Geometry: final body of the model. Coordinates: model frame, mm. A direction names the side the tool comes from. Round coordinates to 2 decimals unless told otherwise and drop trailing zeros. Loops run counter-clockwise (first coordinate to the right, second up) from the corner with the lowest first, then second, coordinate; pieces in that order, holes last. Notation, with made-up numbers: (-10.75, 31) - (22.25, 31) arc R25 cw to (22.25, 49) - close; hole circle Ø7 at (-14, -24). An arc over 180 degrees is marked (long way). Answer as a JSON object with one key per item and string values. Group by question number.
Item 1: Section A-A (x = -18.5). Return the cut outline in (y, z).
Item 2: Section C-C (y = 56). Return the cut outline in (x, z).
Item 3: Line query: line 1 (Z direction, x = -34, y = 81); line 2 (X direction, y = 6, z = 275.5); line 3 (Y direction, x = -4, z = 164.5). Output: solid intervals per line, ascending.
Item 4: Section B-B (z = 112.5). Return the cut outline in (x, y), plus the area to 3 significant figures.
Item 5: Draft query along Z for faces 1 (the face through (-6, 6, 0)), 2 (the face through (0, -7.94, 148)), 3 (the face through (0, 23, 267.65)). Return one class per face: released by +Z, released by -Z, zero draft, split by the parting line, or undercut.
Item 6: First-contact query: pin 1 (21 mm diameter, centred on x = -1.5, y = 23, fed in from -Z); pin 2 (2 mm diameter, centred on x = -12.5, y = 69.5, fed in from -Z); pin 3 (5.5 mm diameter, centred on x = 0, y = 31.94, fed in from -Z); pin 4 (1.2 mm diameter, centred on y = 17.5, z = 54.5, fed in from -X) (3 decimals). Flat tips, straight axial feed; report the tip coordinate or a pass-through.
Item 7: Reachability of faces 4 (the face through (0, 23, 51.38)), 5 (the face through (-6, -6, 0)), 6 (the face through (6, -6, 376)), 7 (the face through (0, 23, 174.38)) from +Z, -Z, +X, -X, +Y, -Y: full face, straight path, thin tool, end or side. Return the list, or none.
```python
from build123d import *

# Parameters (mm, degrees)
CROQUIS2_W              = 15.88
CROQUIS2_H              = 15.88
SALIENTE_EXTRUIR1_DEPTH = 300
CROQUIS3_R              = 7.94
SALIENTE_EXTRUIR2_DEPTH = 50
SALIENTE_EXTRUIR3_START = 50
CROQUIS5_R              = 7.94
SALIENTE_EXTRUIR3_DEPTH = 50
CROQUIS6_W              = 19.05
CROQUIS6_H              = 4
CROQUIS6_H_2            = 3.052323646
SALIENTE_EXTRUIR4_DEPTH = 30
CORTAR_EXTRUIR1_REACH   = 303.171
CROQUIS7_R              = 3
CROQUIS8_R              = 7.94
SALIENTE_EXTRUIR5_DEPTH = 30
CROQUIS9_R              = 15.735705631
SALIENTE_EXTRUIR6_DEPTH = 4


with BuildPart() as part:
    # Croquis2 → Saliente-Extruir1 (new body)
    with BuildSketch(Plane.XY):
        Rectangle(CROQUIS2_W, CROQUIS2_H)
    extrude(amount=SALIENTE_EXTRUIR1_DEPTH)

    # Croquis3 → Saliente-Extruir2 (add)
    with BuildSketch(Plane.XY.offset(300)):
        Circle(CROQUIS3_R)
    extrude(amount=SALIENTE_EXTRUIR2_DEPTH)

    # Croquis5 → Saliente-Extruir3 (add)
    with BuildSketch(Plane(origin=(0, 0, 0), x_dir=(-1, 0, 0), z_dir=(0, 0, -1)).offset(SALIENTE_EXTRUIR3_START)):
        with Locations(Location((0, 0, 0), (0, 0, 180))):
            Circle(CROQUIS5_R)
    extrude(amount=-SALIENTE_EXTRUIR3_DEPTH)

    # Croquis6 → Saliente-Extruir4 (add)
    with BuildSketch(Plane(origin=(0, 7.94, 0), x_dir=(1, 0, 0), z_dir=(0, 1, 0))):
        with Locations((0, -269.65)):
            Rectangle(CROQUIS6_W, CROQUIS6_H)
        with Locations((0, -260.65)):
            Rectangle(CROQUIS6_W, CROQUIS6_H_2)
        with Locations((0, -172.38)):
            Rectangle(CROQUIS6_W, CROQUIS6_H)
        with Locations((0, -163.38)):
            Rectangle(CROQUIS6_W, CROQUIS6_H)
        with Locations((0, -62.38)):
            Rectangle(CROQUIS6_W, CROQUIS6_H)
        with Locations((0, -53.38)):
            Rectangle(CROQUIS6_W, CROQUIS6_H)
    extrude(amount=SALIENTE_EXTRUIR4_DEPTH)

    # Cortar-Extruir1: up to this face of the body (flat: up to its plane)
    cortar_extruir1_end = Plane(part.part.faces().sort_by_distance((0, 22.94, 271.65))[0])
    # Croquis7 → Cortar-Extruir1 (cut, up to the picked face)
    with BuildSketch(Plane(origin=(0, 0, 51.38), x_dir=(-1, 0, 0), z_dir=(0, 0, -1)), mode=Mode.PRIVATE) as cortar_extruir1_sk1:
        with Locations((0, 31.94)):
            Circle(CROQUIS7_R)
    cortar_extruir1_tool1 = split(extrude(cortar_extruir1_sk1.sketch, amount=-CORTAR_EXTRUIR1_REACH, mode=Mode.PRIVATE), bisect_by=cortar_extruir1_end, keep=Keep.BOTH, mode=Mode.PRIVATE)
    add(cortar_extruir1_tool1.solids().sort_by(Axis((0, 31.94, 51.38), (0, 0, 1)))[0], mode=Mode.SUBTRACT)

    # Croquis8 → Saliente-Extruir5 (add)
    with BuildSketch(Plane.XY.offset(350)):
        Circle(CROQUIS8_R)
    extrude(amount=SALIENTE_EXTRUIR5_DEPTH)

    # Croquis9 → Saliente-Extruir6 (add)
    with BuildSketch(Plane.XY.offset(380)):
        with BuildLine():
            Line((-7.94, 7.94), (-7.94, 27.049213062))
            Line((-7.94, 27.049213062), (-7.94, 63.465360978))
            Line((-7.94, 63.465360978), (-22.419294846, 63.465360978))
            ThreePointArc((-22.419294846, 63.465360978), (-33.025896564, 67.85875926), (-37.419294846, 78.465360978))
            Line((-37.419294846, 78.465360978), (-37.419294846, 88.478483412))
            ThreePointArc((-37.419294846, 88.478483412), (-33.025896564, 99.085085129), (-22.419294846, 103.478483412))
            Line((-22.419294846, 103.478483412), (-7.06, 103.478483412))
            ThreePointArc((-7.06, 103.478483412), (3.546601718, 99.085085129), (7.94, 88.478483412))
            Line((7.94, 88.478483412), (7.94, 63.465360978))
            Line((7.94, 63.465360978), (7.94, 7.94))
            Line((7.94, 7.94), (7.94, -7.94))
            Line((7.94, -7.94), (-7.94, -7.94))
            Line((-7.94, -7.94), (-7.94, 7.94))
        make_face()
        with Locations((-14.739647423, 83.471922195)):
            Circle(CROQUIS9_R, mode=Mode.SUBTRACT)
    extrude(amount=-SALIENTE_EXTRUIR6_DEPTH)


solid = part.part
```
Values:
{
 "1": {"outline": "(63.47, 376) - (68.19, 376) - (68.19, 380) - (63.47, 380) - close; (98.75, 376) - (103.48, 376) - (103.48, 380) - (98.75, 380) - close"},
 "2": {"outline": "(-7.94, 376) - (7.94, 376) - (7.94, 380) - (-7.94, 380) - close"},
 "3": {"line 1": "z = 376 to 380", "line 2": "x = -7.94 to 7.94", "line 3": "y = -7.94 to 37.94"},
 "4": {"outline": "(-7.94, -7.94) - (7.94, -7.94) - (7.94, 7.94) - (-7.94, 7.94) - close", "area": "252 mm^2"},
 "5": {"face 1": "released by -Z", "face 2": "zero draft", "face 3": "undercut"},
 "6": {"pin 1": "stops at z = 51.38", "pin 2": "passes through", "pin 3": "stops at z = 376", "pin 4": "stops at x = -9.525"},
 "7": {"face 4": "-Z, +X, -X, +Y", "face 5": "-Z, -X, -Y", "face 6": "+X, -Y", "face 7": "+X, -X, +Y"}
}
